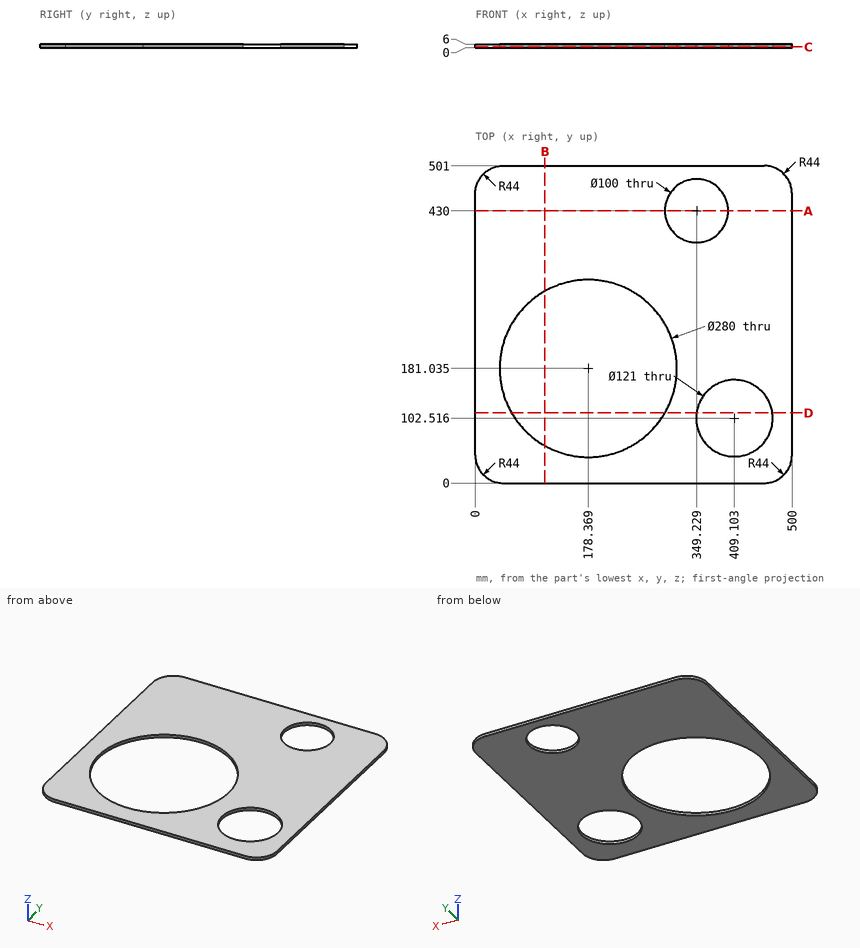
Input: dimensioned drawing with shaded views. Units: mm. Origin: part minimum x, y, z. Coordinates: 2 decimals unless noted, no trailing zeros. Loops run counter-clockwise (first coordinate to the right, second up) from the corner with the lowest first, then second, coordinate; pieces in that order, holes last. Notation, with made-up numbers: (19, 81) - (33, 81) arc R20 ccw to (33, 117) - close; hole circle Ø4 at (-18, 67.5). An arc over 180 degrees is marked (long way). One line per question, with ' | ' between items. Start each with the question number.
(1) Cut plane B-B on x = 110. Output: boundary loops of the cut face in (y, z) (1 decimal).
(2) Cut plane C-C on z = 1.45. Output: boundary loops of the cut face in (x, y) (1 decimal), and give its area (3 significant figures).
(3) Cut plane A-A on y = 430. Output: boundary loops of the cut face in (x, z).
(4) Ray query, L1, parallel to Y at x = 374.5, z = 1.7 (1 decimal); L2, parallel to X at y = 95, z = 3.05 (1 decimal); L3, parallel to Y at x = 406, z = 1.85 (1 decimal). Return the intervals inside material, ascending. Write a range as from..to.
(5) Cut plane D-D on y = 111. Output: boundary loops of the cut face in (x, z) (1 decimal).
Here are the results:
1) outline: (0, 0) - (58.9, 0) - (58.9, 6) - (0, 6) - close; (303.2, 0) - (501, 0) - (501, 6) - (303.2, 6) - close
2) outline: (0, 44) arc R44 ccw to (44, 0) - (456, 0) arc R44 ccw to (500, 44) - (500, 457) arc R44 ccw to (456, 501) - (44, 501) arc R44 ccw to (0, 457) - close; hole circle Ø280 at (178.4, 181); hole circle Ø100 at (349.2, 430); hole circle Ø121 at (409.1, 102.5) | area: 168,000 mm²
3) outline: (0, 0) - (299.23, 0) - (299.23, 6) - (0, 6) - close; (399.23, 0) - (500, 0) - (500, 6) - (399.23, 6) - close
4) L1: 0..52.9, 152.1..386.9, 473.1..501 | L2: 0..67.9, 288.8..349.1, 469.1..500 | L3: 0..42.1, 162.9..501
5) outline: (0, 0) - (57.1, 0) - (57.1, 6) - (0, 6) - close; (299.6, 0) - (349.2, 0) - (349.2, 6) - (299.6, 6) - close; (469, 0) - (500, 0) - (500, 6) - (469, 6) - close
